Could you check a few things on this model? Use its own coordinates, in mm. Face numbers are marked on the shaded views. Round coordinates to 2 decimals unless told otherwise and drop trailing zeros. Loops run counter-clockwise (first coordinate to the right, second up) from the corner with the lowest first, then second, coordinate; pieces in that order, holes last. Notation, with made-up numbers: (75, 2.25) - (109, 2.25) arc R33 ccw to (109, 34.25) - close; hole circle Ø7 at (11, -21.75). An arc over 180 degrees is marked (long way). Answer as CSV lines item,"result". Start each with the question number.
1) Suppose I cut it at B-B, the plane y = -3. Count the separate pieces of the cut face and the enclosed holes in it, then the cut area to 3 significant figures.
2) Please list where these lines run through material, in increasing order: line 1 along X through (y, z) = (14, 1.95) (3 decimals); line 2 along X through (y, z) = (-9, 4.5); line 3 along Y through (x, z) = (-17.5, 2.65).
3) I'm going to push flat-ended pins straight in: pin 1 Ø5 at (x, y) = (31.5, -5) entering from +Z; pin 2 Ø4 at (x, y) = (-36.375, -20.75) entering from +Z; pin 3 Ø0.9 at (y, z) = (-5, 1) entering from -X (3 decimals). Where does each tip first touch, or does it pass through?
4) Suppose I cut it at A-A, the plane z = 2.2. Write out the boundary of the cut face in (x, y) (3 decimals), then the cut area to 3 significant figures.
5) We'd pull the mould along X, two halves only. Please class the marked faces 1 and 2: pulls with the +X half, pulls with the -X half, needs draft (parallel to the pull), parting line crosses it, or undercut.
6) Suppose I cut it at D-D, the plane x = 33. Write out the boundary of the cut face in (y, z), then the cut area to 4 significant figures.
```python
from build123d import *

# Parameters (mm, degrees)
ESBO_O1_W                = 68.75
ESBO_O1_H                = 49.5
RESSALTO_EXTRUS_O1_DEPTH = 5
ESBO_O2_W                = 60.75
ESBO_O2_H                = 41
CORTE_EXTRUS_O1_DEPTH    = 3
ESBO_O3_R                = 1.8
RESSALTO_EXTRUS_O2_DEPTH = 3
ESBO_O4_W                = 68.75
ESBO_O4_H                = 49.5
ESBO_O4_W_2              = 63.75
ESBO_O4_H_2              = 44.5
CORTE_EXTRUS_O2_DEPTH    = 2
CHANFRO1_SIZE            = 2
ESBO_O6_R                = 10.499996118
ESBO_O6_R_2              = 12.499999064
CORTE_EXTRUS_O4_DEPTH    = 48.620406603


with BuildPart() as part:
    # Esboço1 → Ressalto-extrusão1 (new body)
    with BuildSketch(Plane.XY):
        Rectangle(ESBO_O1_W, ESBO_O1_H)
    extrude(amount=RESSALTO_EXTRUS_O1_DEPTH)

    # Esboço2 → Corte-extrusão1 (cut)
    with BuildSketch(Plane(origin=(0, 0, 0), x_dir=(-1, 0, 0), z_dir=(0, 0, -1))):
        Rectangle(ESBO_O2_W, ESBO_O2_H)
    extrude(amount=-CORTE_EXTRUS_O1_DEPTH, mode=Mode.SUBTRACT)

    # Esboço3 → Ressalto-extrusão2 (add)
    # profile 1 of 4: a face of its own
    with BuildSketch(Plane(origin=(0, 0, 0), x_dir=(-1, 0, 0), z_dir=(0, 0, -1))):
        with BuildLine():
            Line((-36.375, 24.75), (-34.375, 24.75))
            Line((-34.375, 24.75), (-34.375, 16.75))
            Line((-34.375, 16.75), (-36.375, 16.75))
            ThreePointArc((-36.375, 16.75), (-40.375, 20.75), (-36.375, 24.75))
        make_face()
        with Locations((-36.375, 20.75)):
            Circle(ESBO_O3_R, mode=Mode.SUBTRACT)
    # profile 2 of 4: a face of its own
    with BuildSketch(Plane(origin=(0, 0, 0), x_dir=(-1, 0, 0), z_dir=(0, 0, -1))):
        with BuildLine():
            Line((34.375, 16.75), (36.375, 16.75))
            ThreePointArc((36.375, 16.75), (40.375, 20.75), (36.375, 24.75))
            Line((36.375, 24.75), (34.375, 24.75))
            Line((34.375, 24.75), (34.375, 16.75))
        make_face()
        with Locations(Location((36.375, 20.75, 0), (0, 0, 180))):
            Circle(ESBO_O3_R, mode=Mode.SUBTRACT)
    # profile 3 of 4: a face of its own
    with BuildSketch(Plane(origin=(0, 0, 0), x_dir=(-1, 0, 0), z_dir=(0, 0, -1))):
        with BuildLine():
            Line((36.375, -24.75), (34.375, -24.75))
            Line((34.375, -24.75), (34.375, -16.75))
            Line((34.375, -16.75), (36.375, -16.75))
            ThreePointArc((36.375, -16.75), (40.375, -20.75), (36.375, -24.75))
        make_face()
        with Locations((36.375, -20.75)):
            Circle(ESBO_O3_R, mode=Mode.SUBTRACT)
    # profile 4 of 4: a face of its own
    with BuildSketch(Plane(origin=(0, 0, 0), x_dir=(-1, 0, 0), z_dir=(0, 0, -1))):
        with BuildLine():
            Line((-34.375, -16.75), (-36.375, -16.75))
            ThreePointArc((-36.375, -16.75), (-40.375, -20.75), (-36.375, -24.75))
            Line((-36.375, -24.75), (-34.375, -24.75))
            Line((-34.375, -24.75), (-34.375, -16.75))
        make_face()
        with Locations(Location((-36.375, -20.75, 0), (0, 0, 180))):
            Circle(ESBO_O3_R, mode=Mode.SUBTRACT)
    extrude(amount=-RESSALTO_EXTRUS_O2_DEPTH)

    # Esboço4 → Corte-extrusão2 (cut)
    with BuildSketch(Plane.XY.offset(5)):
        Rectangle(ESBO_O4_W, ESBO_O4_H)
        Rectangle(ESBO_O4_W_2, ESBO_O4_H_2, mode=Mode.SUBTRACT)
    extrude(amount=-CORTE_EXTRUS_O2_DEPTH, mode=Mode.SUBTRACT)

    # Chanfro1
    chanfro1_edges = [part.edges().sort_by_distance(p)[0] for p in [
        (31.875, 0, 5),
        (0, -22.25, 5),
        (-31.875, 0, 5),
        (0, 22.25, 5),
    ]]
    chamfer(chanfro1_edges, length=CHANFRO1_SIZE - 0.0001)  # a hair under: the kernel refuses the full size

    # Esboço6 → Corte-extrusão4 (cut, through all)
    with BuildSketch(Plane.XY.offset(5)):
        with Locations((-15.805529429, 0.050006416)):
            Circle(ESBO_O6_R)
        with Locations((11.094471539, 0.049998219)):
            Circle(ESBO_O6_R_2)
    extrude(amount=-CORTE_EXTRUS_O4_DEPTH, mode=Mode.SUBTRACT)


solid = part.part
```
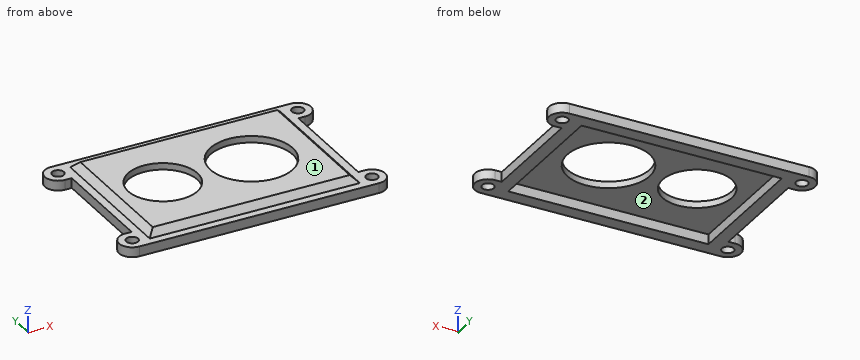
Filled sheet:
1,separate pieces,"3"
1,enclosed holes,"0"
1,area,"58.8 mm²"
2,line 1,"-34.375 to -30.375, 30.375 to 34.375"
2,line 2,"-30.38 to -21.13, -10.48 to 2.47, 19.72 to 30.38"
2,line 3,"-24.75 to -20.5, 20.5 to 24.75"
3,pin 1,"z = 5"
3,pin 2,"z = 3"
3,pin 3,"x = -34.375"
4,outline,"(-36.375, -24.75) - (36.375, -24.75) arc R4 ccw to (36.375, -16.75) - (34.375, -16.75) - (34.375, 16.75) - (36.375, 16.75) arc R4 ccw to (36.375, 24.75) - (-36.375, 24.75) arc R4 ccw to (-36.375, 16.75) - (-34.375, 16.75) - (-34.375, -16.75) - (-36.375, -16.75) arc R4 ccw to start; hole circle Ø3.6 at (-36.375, -20.75); hole circle Ø3.6 at (-36.375, 20.75); hole (-30.375, -20.5) - (30.375, -20.5) - (30.375, 20.5) - (-30.375, 20.5) - close; hole circle Ø3.6 at (36.375, -20.75); hole circle Ø3.6 at (36.375, 20.75)"
4,area,"1,040 mm²"
5,face 1,"needs draft"
5,face 2,"undercut"
6,outline,"(-24.75, 0) - (24.75, 0) - (24.75, 3) - (-24.75, 3) - close"
6,area,"148.5 mm²"
